```python
from build123d import *

# Parameters (mm, degrees)
BOSS_EXTRUDE1_DEPTH                             = 47.371
SKETCH2_W                                       = 6.858
SKETCH2_H                                       = 3.429
CUT_EXTRUDE1_DEPTH                              = 49.438972089
SKETCH3_W                                       = 4.064
SKETCH3_H                                       = 47.371
BOSS_EXTRUDE2_DEPTH                             = 7.366
SKETCH4_W                                       = 6.858
SKETCH4_H                                       = 3.429
CUT_EXTRUDE2_DEPTH                              = 50.110425431
SKETCH5_W                                       = 4.064
SKETCH5_H                                       = 47.371
BOSS_EXTRUDE3_DEPTH                             = 7.366
F_3_CLEARANCE_HOLE1_D                           = 2.7686
CBORE_FOR_10_BUTTON_HEAD_CAP_SCREW1_D           = 5.1054
CBORE_FOR_10_BUTTON_HEAD_CAP_SCREW1_CBORE_D     = 9.92124
CBORE_FOR_10_BUTTON_HEAD_CAP_SCREW1_CBORE_DEPTH = 3.2004
FILLET1_R                                       = 1.27
FILLET3_R                                       = 1.27
FILLET5_R                                       = 1.27


with BuildPart() as part:
    # Sketch1 → Boss-Extrude1 (new body)
    with BuildSketch(Plane.XY.offset(23.6855)):
        Polygon((3.302, 6.35), (-4.064, 6.35), (-4.064, -6.35), (3.302, -6.35), (7.874, -2.54), (7.874, 2.54), align=None)
    extrude(amount=-BOSS_EXTRUDE1_DEPTH)

    # Sketch2 → Cut-Extrude1 (cut, through all)
    with BuildSketch(Plane.XY.offset(23.6855)):
        with Locations((-0.635, 4.6355)):
            Rectangle(SKETCH2_W, SKETCH2_H)
    extrude(amount=-CUT_EXTRUDE1_DEPTH, mode=Mode.SUBTRACT)

    # Sketch3 → Boss-Extrude2 (add)
    with BuildSketch(Plane(origin=(0, 2.921, 0), x_dir=(-1, 0, 0), z_dir=(0, 1, 0))):
        with Locations((2.032, 0)):
            Rectangle(SKETCH3_W, SKETCH3_H)
    extrude(amount=BOSS_EXTRUDE2_DEPTH)

    # Sketch4 → Cut-Extrude2 (cut, through all)
    with BuildSketch(Plane.XY.offset(23.6855)):
        with Locations((-0.635, -4.6355)):
            Rectangle(SKETCH4_W, SKETCH4_H)
    extrude(amount=-CUT_EXTRUDE2_DEPTH, mode=Mode.SUBTRACT)

    # Sketch5 → Boss-Extrude3 (add)
    with BuildSketch(Plane.XZ.offset(2.921)):
        with Locations((-2.032, 0)):
            Rectangle(SKETCH5_W, SKETCH5_H)
    extrude(amount=BOSS_EXTRUDE3_DEPTH)

    # #3 Clearance Hole1 (through all)
    with Locations(Plane.ZY.offset(4.064)):
        with Locations((12.7, 0), (-12.7, 0)):
            Hole(F_3_CLEARANCE_HOLE1_D / 2)

    # CBORE for #10 Button Head Cap Screw1 (through all)
    with Locations(Plane(origin=(7.874, 0, 0), x_dir=(0, 0, -1), z_dir=(1, 0, 0))):
        with Locations((-12.7, 0), (12.7, 0)):
            CounterBoreHole(CBORE_FOR_10_BUTTON_HEAD_CAP_SCREW1_D / 2, CBORE_FOR_10_BUTTON_HEAD_CAP_SCREW1_CBORE_D / 2, CBORE_FOR_10_BUTTON_HEAD_CAP_SCREW1_CBORE_DEPTH)

    # Fillet1
    fillet1_edges = [part.edges().sort_by_distance(p)[0] for p in [
        (7.874, -2.54, 20.323251747),
        (7.874, -2.54, -20.323251747),
        (7.874, -2.54, 0),
        (7.874, 2.54, 20.323251747),
        (7.874, 2.54, 0),
        (7.874, 2.54, -20.323251747),
    ]]
    fillet(fillet1_edges, radius=FILLET1_R)

    # Fillet3
    # the kernel refuses this fillet: 1.27 mm, written as the material it takes off along each edge
    with BuildSketch(Plane(origin=(0.862897437, -8.382585469, -23.6855), x_dir=(0, 0, 1), z_dir=(0.7682212795973759, 0.6401843996644799, 0)), Plane(origin=(7.417034188, 2.920804844, -23.6855), x_dir=(0, 0, 1), z_dir=(-0.7682212795973759, 0.6401843996644799, 0))) as fillet3_piece_1:
        with BuildLine():
            CenterArc((FILLET3_R, -FILLET3_R), FILLET3_R, 90, 90)
            Line((0, -FILLET3_R), (0, 0))
            Line((0, 0), (FILLET3_R, 0))
        make_face()
    extrude(amount=8.531574072, mode=Mode.SUBTRACT)
    with BuildSketch(Plane(origin=(6.604, -1.945163819, -23.6855), x_dir=(0.6401843996644796, -0.7682212795973762, 0), z_dir=(-0.7682212795973762, -0.6401843996644796, 0))) as fillet3_piece_2:
        with BuildLine():
            CenterArc((1.27 - FILLET3_R, FILLET3_R), FILLET3_R, 270, 90)
            Line((1.27, FILLET3_R), (1.27, 0))
            Line((1.27, 0), (1.27 - FILLET3_R, 0))
        make_face()
    revolve(axis=Axis((6.604, -1.945163819, -23.6855), (0, 0, 1)), revolution_arc=50.194428908, mode=Mode.SUBTRACT)
    with BuildSketch(Plane(origin=(6.604, 1.945163819, -23.6855), x_dir=(0.6401843996644799, 0.7682212795973757, 0), z_dir=(-0.7682212795973757, 0.6401843996644799, 0))) as fillet3_piece_3:
        with BuildLine():
            CenterArc((1.27 - FILLET3_R, -FILLET3_R), FILLET3_R, 0, 90)
            Line((1.27, -FILLET3_R), (1.27, 0))
            Line((1.27, 0), (1.27 - FILLET3_R, 0))
        make_face()
    revolve(axis=Axis((6.604, 1.945163819, -23.6855), (0, 0, -1)), revolution_arc=50.194428908, mode=Mode.SUBTRACT)
    with BuildSketch(Plane(origin=(2.794, -2.921, -23.6855), x_dir=(0, 0, 1), z_dir=(-1, 0, 0)), Plane(origin=(0, 2.921, -23.6855), x_dir=(0, 0, 1), z_dir=(1, 0, 0))) as fillet3_piece_4:
        with BuildLine():
            CenterArc((FILLET3_R, FILLET3_R), FILLET3_R, 180, 90)
            Line((0, FILLET3_R), (0, 0))
            Line((0, 0), (FILLET3_R, 0))
        make_face()
    extrude(amount=2.794, mode=Mode.SUBTRACT)
    with BuildSketch(Plane(origin=(2.794, 2.921, -23.6855), x_dir=(0, 0, 1), z_dir=(0, 1, 0)), Plane(origin=(2.794, -9.525, -23.6855), x_dir=(0, 0, 1), z_dir=(0, 1, 0))) as fillet3_piece_5:
        with BuildLine():
            CenterArc((FILLET3_R, FILLET3_R), FILLET3_R, 180, 90)
            Line((0, FILLET3_R), (0, 0))
            Line((0, 0), (FILLET3_R, 0))
        make_face()
    extrude(amount=6.604, mode=Mode.SUBTRACT)
    with BuildSketch(Plane(origin=(7.874, -1.945163819, -23.6855), x_dir=(-1, 0, 0), z_dir=(0, 1, 0))) as fillet3_piece_6:
        with BuildLine():
            CenterArc((FILLET3_R, FILLET3_R), FILLET3_R, 180, 90)
            Line((0, FILLET3_R), (0, 0))
            Line((0, 0), (FILLET3_R, 0))
        make_face()
    extrude(amount=3.890327637, mode=Mode.SUBTRACT)
    with BuildSketch(Plane(origin=(2.794, -9.525, -23.6855), x_dir=(0, 0, 1), z_dir=(0, 1, 0))) as fillet3_piece_7a_section:
        with BuildLine():
            CenterArc((FILLET3_R, FILLET3_R), FILLET3_R, 180, 90)
            Line((0, FILLET3_R), (0, 0))
            Line((0, 0), (FILLET3_R, 0))
        make_face()
    fillet3_piece_7a = extrude(amount=9.779, mode=Mode.PRIVATE)
    fillet3_piece_7a = split(fillet3_piece_7a, bisect_by=Plane(origin=(3.081521795, -2.921, -23.397978205), z_dir=(0, 1, 0)), keep=Keep.TOP, mode=Mode.PRIVATE)
    with BuildSketch(Plane(origin=(5.969, -2.921, -23.6855), x_dir=(0, 0, 1), z_dir=(-1, 0, 0))) as fillet3_piece_7b_section:
        with BuildLine():
            CenterArc((FILLET3_R, FILLET3_R), FILLET3_R, 180, 90)
            Line((0, FILLET3_R), (0, 0))
            Line((0, 0), (FILLET3_R, 0))
        make_face()
    fillet3_piece_7b = extrude(amount=5.969, mode=Mode.PRIVATE)
    fillet3_piece_7b = split(fillet3_piece_7b, bisect_by=Plane(origin=(2.794, -2.633478205, -23.397978205), z_dir=(1, 0, 0)), keep=Keep.TOP, mode=Mode.PRIVATE)
    fillet3_piece_7 = fillet3_piece_7a & fillet3_piece_7b
    add(fillet3_piece_7, mode=Mode.SUBTRACT)
    with BuildSketch(Plane(origin=(2.794, -0.254, -23.6855), x_dir=(0, 0, 1), z_dir=(0, 1, 0))) as fillet3_piece_8a_section:
        with BuildLine():
            CenterArc((FILLET3_R, FILLET3_R), FILLET3_R, 180, 90)
            Line((0, FILLET3_R), (0, 0))
            Line((0, 0), (FILLET3_R, 0))
        make_face()
    fillet3_piece_8a = extrude(amount=9.779, mode=Mode.PRIVATE)
    fillet3_piece_8a = split(fillet3_piece_8a, bisect_by=Plane(origin=(3.081521795, 2.921, -23.397978205), z_dir=(0, -1, 0)), keep=Keep.TOP, mode=Mode.PRIVATE)
    with BuildSketch(Plane(origin=(0, 2.921, -23.6855), x_dir=(0, 0, 1), z_dir=(1, 0, 0))) as fillet3_piece_8b_section:
        with BuildLine():
            CenterArc((FILLET3_R, FILLET3_R), FILLET3_R, 180, 90)
            Line((0, FILLET3_R), (0, 0))
            Line((0, 0), (FILLET3_R, 0))
        make_face()
    fillet3_piece_8b = extrude(amount=5.969, mode=Mode.PRIVATE)
    fillet3_piece_8b = split(fillet3_piece_8b, bisect_by=Plane(origin=(2.794, 2.633478205, -23.397978205), z_dir=(1, 0, 0)), keep=Keep.TOP, mode=Mode.PRIVATE)
    fillet3_piece_8 = fillet3_piece_8a & fillet3_piece_8b
    add(fillet3_piece_8, mode=Mode.SUBTRACT)

    # Fillet5
    # the kernel refuses this fillet: 1.27 mm, written as the material it takes off along each edge
    with BuildSketch(Plane(origin=(0.862897437, -8.382585469, 23.6855), x_dir=(-0.6401843996644799, 0.7682212795973759, 0), z_dir=(0.7682212795973759, 0.6401843996644799, 0)), Plane(origin=(7.417034188, 2.920804844, 23.6855), x_dir=(-0.6401843996644799, -0.7682212795973759, 0), z_dir=(-0.7682212795973759, 0.6401843996644799, 0))) as fillet5_piece_1:
        with BuildLine():
            CenterArc((FILLET5_R, -FILLET5_R), FILLET5_R, 90, 90)
            Line((0, -FILLET5_R), (0, 0))
            Line((0, 0), (FILLET5_R, 0))
        make_face()
    extrude(amount=8.531574072, mode=Mode.SUBTRACT)
    with BuildSketch(Plane(origin=(6.604, -1.945163819, 23.6855), x_dir=(1, 0, 0), z_dir=(0, 1, 0))) as fillet5_piece_2:
        with BuildLine():
            CenterArc((1.27 - FILLET5_R, FILLET5_R), FILLET5_R, 270, 90)
            Line((1.27, FILLET5_R), (1.27, 0))
            Line((1.27, 0), (1.27 - FILLET5_R, 0))
        make_face()
    revolve(axis=Axis((6.604, -1.945163819, 23.6855), (0, 0, -1)), revolution_arc=50.194428908, mode=Mode.SUBTRACT)
    with BuildSketch(Plane(origin=(6.604, 1.945163819, 23.6855), x_dir=(0.6401843996644799, 0.7682212795973757, 0), z_dir=(-0.7682212795973757, 0.6401843996644799, 0))) as fillet5_piece_3:
        with BuildLine():
            CenterArc((1.27 - FILLET5_R, FILLET5_R), FILLET5_R, 270, 90)
            Line((1.27, FILLET5_R), (1.27, 0))
            Line((1.27, 0), (1.27 - FILLET5_R, 0))
        make_face()
    revolve(axis=Axis((6.604, 1.945163819, 23.6855), (0, 0, -1)), revolution_arc=50.194428908, mode=Mode.SUBTRACT)
    with BuildSketch(Plane(origin=(2.794, 2.921, 23.6855), x_dir=(1, 0, 0), z_dir=(0, 1, 0)), Plane(origin=(2.794, -9.525, 23.6855), x_dir=(1, 0, 0), z_dir=(0, 1, 0))) as fillet5_piece_4:
        with BuildLine():
            CenterArc((FILLET5_R, FILLET5_R), FILLET5_R, 180, 90)
            Line((0, FILLET5_R), (0, 0))
            Line((0, 0), (FILLET5_R, 0))
        make_face()
    extrude(amount=6.604, mode=Mode.SUBTRACT)
    with BuildSketch(Plane(origin=(0, 2.921, 23.6855), x_dir=(0, -1, 0), z_dir=(1, 0, 0)), Plane(origin=(2.794, -2.921, 23.6855), x_dir=(0, 1, 0), z_dir=(-1, 0, 0))) as fillet5_piece_5:
        with BuildLine():
            CenterArc((FILLET5_R, FILLET5_R), FILLET5_R, 180, 90)
            Line((0, FILLET5_R), (0, 0))
            Line((0, 0), (FILLET5_R, 0))
        make_face()
    extrude(amount=2.794, mode=Mode.SUBTRACT)
    with BuildSketch(Plane(origin=(7.874, -1.945163819, 23.6855), x_dir=(-1, 0, 0), z_dir=(0, 1, 0))) as fillet5_piece_6:
        with BuildLine():
            CenterArc((FILLET5_R, -FILLET5_R), FILLET5_R, 90, 90)
            Line((0, -FILLET5_R), (0, 0))
            Line((0, 0), (FILLET5_R, 0))
        make_face()
    extrude(amount=3.890327637, mode=Mode.SUBTRACT)
    with BuildSketch(Plane(origin=(2.794, -0.254, 23.6855), x_dir=(1, 0, 0), z_dir=(0, 1, 0))) as fillet5_piece_7a_section:
        with BuildLine():
            CenterArc((FILLET5_R, FILLET5_R), FILLET5_R, 180, 90)
            Line((0, FILLET5_R), (0, 0))
            Line((0, 0), (FILLET5_R, 0))
        make_face()
    fillet5_piece_7a = extrude(amount=9.779, mode=Mode.PRIVATE)
    fillet5_piece_7a = split(fillet5_piece_7a, bisect_by=Plane(origin=(3.081521795, 2.921, 23.397978205), z_dir=(0, -1, 0)), keep=Keep.TOP, mode=Mode.PRIVATE)
    with BuildSketch(Plane(origin=(0, 2.921, 23.6855), x_dir=(0, -1, 0), z_dir=(1, 0, 0))) as fillet5_piece_7b_section:
        with BuildLine():
            CenterArc((FILLET5_R, FILLET5_R), FILLET5_R, 180, 90)
            Line((0, FILLET5_R), (0, 0))
            Line((0, 0), (FILLET5_R, 0))
        make_face()
    fillet5_piece_7b = extrude(amount=5.969, mode=Mode.PRIVATE)
    fillet5_piece_7b = split(fillet5_piece_7b, bisect_by=Plane(origin=(2.794, 2.633478205, 23.397978205), z_dir=(1, 0, 0)), keep=Keep.TOP, mode=Mode.PRIVATE)
    fillet5_piece_7 = fillet5_piece_7a & fillet5_piece_7b
    add(fillet5_piece_7, mode=Mode.SUBTRACT)
    with BuildSketch(Plane(origin=(2.794, -9.525, 23.6855), x_dir=(1, 0, 0), z_dir=(0, 1, 0))) as fillet5_piece_8a_section:
        with BuildLine():
            CenterArc((FILLET5_R, FILLET5_R), FILLET5_R, 180, 90)
            Line((0, FILLET5_R), (0, 0))
            Line((0, 0), (FILLET5_R, 0))
        make_face()
    fillet5_piece_8a = extrude(amount=9.779, mode=Mode.PRIVATE)
    fillet5_piece_8a = split(fillet5_piece_8a, bisect_by=Plane(origin=(3.081521795, -2.921, 23.397978205), z_dir=(0, 1, 0)), keep=Keep.TOP, mode=Mode.PRIVATE)
    with BuildSketch(Plane(origin=(5.969, -2.921, 23.6855), x_dir=(0, 1, 0), z_dir=(-1, 0, 0))) as fillet5_piece_8b_section:
        with BuildLine():
            CenterArc((FILLET5_R, FILLET5_R), FILLET5_R, 180, 90)
            Line((0, FILLET5_R), (0, 0))
            Line((0, 0), (FILLET5_R, 0))
        make_face()
    fillet5_piece_8b = extrude(amount=5.969, mode=Mode.PRIVATE)
    fillet5_piece_8b = split(fillet5_piece_8b, bisect_by=Plane(origin=(2.794, -2.633478205, 23.397978205), z_dir=(1, 0, 0)), keep=Keep.TOP, mode=Mode.PRIVATE)
    fillet5_piece_8 = fillet5_piece_8a & fillet5_piece_8b
    add(fillet5_piece_8, mode=Mode.SUBTRACT)


solid = part.part
```
The model under review builds one solid part; all positions refer to its coordinate system, in mm. A direction names the side the tool comes from. Give positions to 0.01 mm unless a question says otherwise; leave off trailing zeros. Write each loop counter-clockwise with the first axis right and the second up, starting at its lowest first coordinate (ties: lowest second). Pieces come first, ordered by that corner, then holes. Notation, with made-up numbers: (15.25, 83.25) -> (62.25, 83.25) arc R12 ccw to (62.25, 89.25) -> close; hole circle Ø2 at (-36.75, 68). An arc over 180 degrees is marked (long way). Answer in a Markdown table with one row per item.
1) For L1, parallel to Z at x = 6.65, y = 0; L2, parallel to Y at x = 0.25, z = -12.7; L3, parallel to Y at x = -1.5, z = -12.7, list the stretches that pass through material, from the lowest coordinate up. Write a range as [from, to].
Worked answers:
| item | result |
|---|---|
| L1 | [-23.68, -17.66], [-7.74, 7.74], [17.66, 23.68] |
| L2 | [-2.92, -2.55], [2.55, 2.92] |
| L3 | [-10.29, -2.55], [2.55, 10.29] |
2) Add section D-D on x = -3. State the section outline as (y, z) points, plus the area to 3 significant figures.
Worked answers:
| item | result |
|---|---|
| outline | (-10.29, -23.69) -> (10.29, -23.69) -> (10.29, 23.69) -> (-10.29, 23.69) -> close; hole circle Ø5.11 at (0, -12.7); hole circle Ø5.11 at (0, 12.7) |
| area | 934 mm² |
3) Tool access review of faces 4 (the flat face through (4.674, -2.1, 10.6)), 5 (the flat face through (7.874, 0, 0)), 6 (the cylindrical face through (1.55, 2.56, 23.3)), 7 (the flat face through (2.794, 5, 0)), 8 (the flat face through (4.873, -5.04, 0.314)): name each direction out of +Z, -Z, +X, -X, +Y, -Y from which nothing blocks a thin tool from reaching the whole face with its end or side.
Worked answers:
| item | result |
|---|---|
| face 4 | +X |
| face 5 | +Z, -Z, +X, +Y, -Y |
| face 6 | +Z, +Y |
| face 7 | +Z, -Z, +Y |
| face 8 | +Z, -Z, +X, -Y |
4) Add section A-A on y = 0. State the section outline as (x, z) points, plus the area to 3 significant figures.
Worked answers:
| item | result |
|---|---|
| outline | (-4.06, -23.69) -> (6.6, -23.69) arc R1.27 ccw to (7.87, -22.42) -> (7.87, -17.66) -> (4.67, -17.66) -> (4.67, -15.25) -> (-4.06, -15.25) -> close; (-4.06, -10.15) -> (4.67, -10.15) -> (4.67, -7.74) -> (7.87, -7.74) -> (7.87, 7.74) -> (4.67, 7.74) -> (4.67, 10.15) -> (-4.06, 10.15) -> close; (-4.06, 15.25) -> (4.67, 15.25) -> (4.67, 17.66) -> (7.87, 17.66) -> (7.87, 22.42) arc R1.27 ccw to (6.6, 23.69) -> (-4.06, 23.69) -> close |
| area | 412 mm² |
5) Add section C-C on z = -14. State the section outline as (x, y) points.
Worked answers:
| item | result |
|---|---|
| outline | (-4.06, -10.29) -> (0, -10.29) -> (0, -2.92) -> (2.79, -2.92) -> (2.79, -6.35) -> (3.3, -6.35) -> (5.18, -4.79) -> (4.67, -4.79) -> (4.67, -2.2) -> (-4.06, -2.2) -> close; (-4.06, 2.2) -> (4.67, 2.2) -> (4.67, 4.79) -> (5.18, 4.79) -> (3.3, 6.35) -> (2.79, 6.35) -> (2.79, 2.92) -> (0, 2.92) -> (0, 10.29) -> (-4.06, 10.29) -> close |
6) Clearance check with flat-ended pins moving along their axes: P1, Ø5, axis at y = 1, z = 14, coming from the +X side; P2, Ø4, axis at x = 2.5, z = -17, coming from the +Y side; P3, Ø12, axis at y = -7.5, z = 10.5, coming from the +X side; P4, Ø5, axis at y = 4, z = -12.5, coming from the +X side. State where each tip first meets the part, or that it passes through.
Worked answers:
| item | result |
|---|---|
| P1 | x = 4.67 |
| P2 | y = 6.35 |
| P3 | x = 7.87 |
| P4 | x = 5.92 |
7) Mouldability with a two-part tool opening along Z and no side actions: class faces 1 (the cylindrical face through (5.88, 1.49, 7.97)), 2 (the cylindrical face through (3.156, -4.033, 23.304)), 3 (the flat face through (0, -6, 0)) as +Z half, -Z half, draft (parallel to the pull), parting line (faces both ways), or undercut.
Worked answers:
| item | result |
|---|---|
| face 1 | undercut |
| face 2 | +Z half |
| face 3 | draft |
8) Add section B-B on z = -7. State the section outline as (x, y) points, plus the area to 3 significant figures.
Worked answers:
| item | result |
|---|---|
| outline | (-4.06, -10.29) -> (0, -10.29) -> (0, -2.92) -> (2.79, -2.92) -> (2.79, -6.35) -> (3.3, -6.35) -> (7.42, -2.92) arc R1.27 ccw to (7.87, -1.95) -> (7.87, 1.95) arc R1.27 ccw to (7.42, 2.92) -> (3.3, 6.35) -> (2.79, 6.35) -> (2.79, 2.92) -> (0, 2.92) -> (0, 10.29) -> (-4.06, 10.29) -> close |
| area | 147 mm² |
